from build123d import *

# Parameters (mm, degrees)
M3X0_5_TAPPED_HOLE1_D = 2.5


with BuildPart() as part:
    # Sketch1 → Revolve1 (revolve)
    with BuildSketch(Plane(origin=(0, 0, 0), x_dir=(1, 0, 0), z_dir=(0, 1, 0))):
        Polygon((-1.75, 0), (-10, 0), (-10, 2), (-4.5, 2), (-4.5, 4.5), (-2.75, 4.5), (-2.75, 1), (-1.75, 1), align=None)
    revolve(axis=Axis((0, 0, -13.360266154), (0, 0, 1)))

    # M3x0.5 Tapped Hole1 (through all)
    with Locations(Plane(origin=(0, 0, -2), x_dir=(-1, 0, 0), z_dir=(0, 0, -1))):
        with Locations((0, 7), (7, 0), (0, -7), (-7, 0)):
            Hole(M3X0_5_TAPPED_HOLE1_D / 2)


solid = part.part
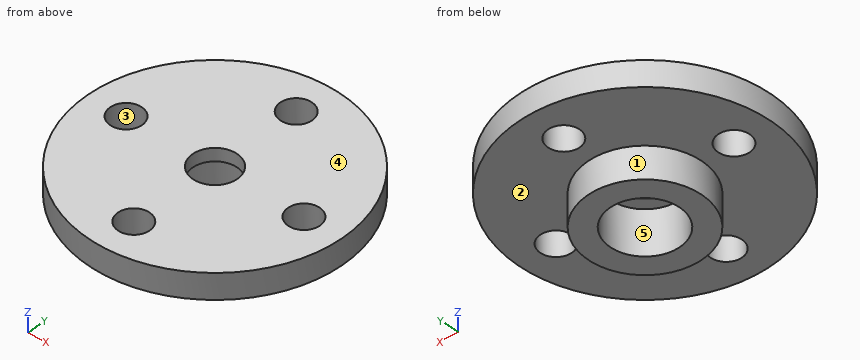
Part model, mm, in its own coordinate system. Face numbers are marked on the shaded views. A direction names the side the tool comes from. Coordinates: 2 decimals unless noted, no trailing zeros. Order: outer loops, then holes, each group sorted by start corner. A loop starts at its lowest first (then second) coordinate and runs counter-clockwise, first axis right, second up. Notation, with made-up numbers: M 89,35 L 110,35 A22 cw 110,56 Z; hole C -39,14.5 d3. An arc over 180 degrees is marked long. One line per question, with ' | ' between items.
Q1. Slice it at A-A (x = 0). Give the cut face in (y, z), and give its area (4 significant figures).
A:
outline: M -10,-2 L -8.25,-2 L -8.25,0 L -10,0 Z; M -5.75,-2 L -4.5,-2 L -4.5,-4.5 L -2.75,-4.5 L -2.75,-1 L -1.75,-1 L -1.75,0 L -5.75,0 Z; M 1.75,-1 L 2.75,-1 L 2.75,-4.5 L 4.5,-4.5 L 4.5,-2 L 5.75,-2 L 5.75,0 L 1.75,0 Z; M 8.25,-2 L 10,-2 L 10,0 L 8.25,0 Z | area: 29.75 mm^2
Q2. Drill centre lines: line 1 (Y direction, x = 0, z = -0.5); line 2 (Y direction, x = 0, z = -1.05); line 3 (X direction, y = 0, z = -2.6). Where is each one in solid material? Low to high.
A:
line 1: y = -10 to -8.25, -5.75 to -1.75, 1.75 to 5.75, 8.25 to 10 | line 2: y = -10 to -8.25, -5.75 to -2.75, 2.75 to 5.75, 8.25 to 10 | line 3: x = -4.5 to -2.75, 2.75 to 4.5
Q3. Two-plate mould, pull along X, no slides. Class the marked faces 1, 2 and 3: +X half, -X half, draft (parallel to the pull), parting line (faces both ways), or undercut.
A:
face 1: parting line | face 2: draft | face 3: undercut
Q4. 3-axis set-ups, long thin cutter, end or side, ignore diameter. For the marked faces 4 and 5: which of +Z, -Z, +X, -X, +Y, -Y reach the whole face in a straight line?
A:
face 4: +Z, +X, -X, +Y, -Y | face 5: -Z
Q5. Slice it at B-B (z = -0.35). Give the cut face in (x, y), and give its area (3 significant figures).
A:
outline: C 0,0 d20; hole C -7,0 d2.5; hole C 0,0 d3.5; hole C 0,-7 d2.5; hole C 0,7 d2.5; hole C 7,0 d2.5 | area: 285 mm^2
Q6. Slice it at D-D (y = -7). Give the cut face in (x, z), and give its area (3 significant figures).
A:
outline: M -7.14,-2 L -1.25,-2 L -1.25,0 L -7.14,0 Z; M 1.25,-2 L 7.14,-2 L 7.14,0 L 1.25,0 Z | area: 23.6 mm^2
Q7. Pin check, flat tips, straight feed: P1, Ø3, axis at x = 7, y = -3.5, coming from the -Z side; P2, Ø1.5, axis at x = -3, z = -1, coming from the -Y side; P3, Ø4.5, axis at x = 0, y = 0, coming from the -Z side. Stop position of each tip, or through.
A:
P1: stops at z = -2 | P2: stops at y = -9.74 | P3: stops at z = -1
